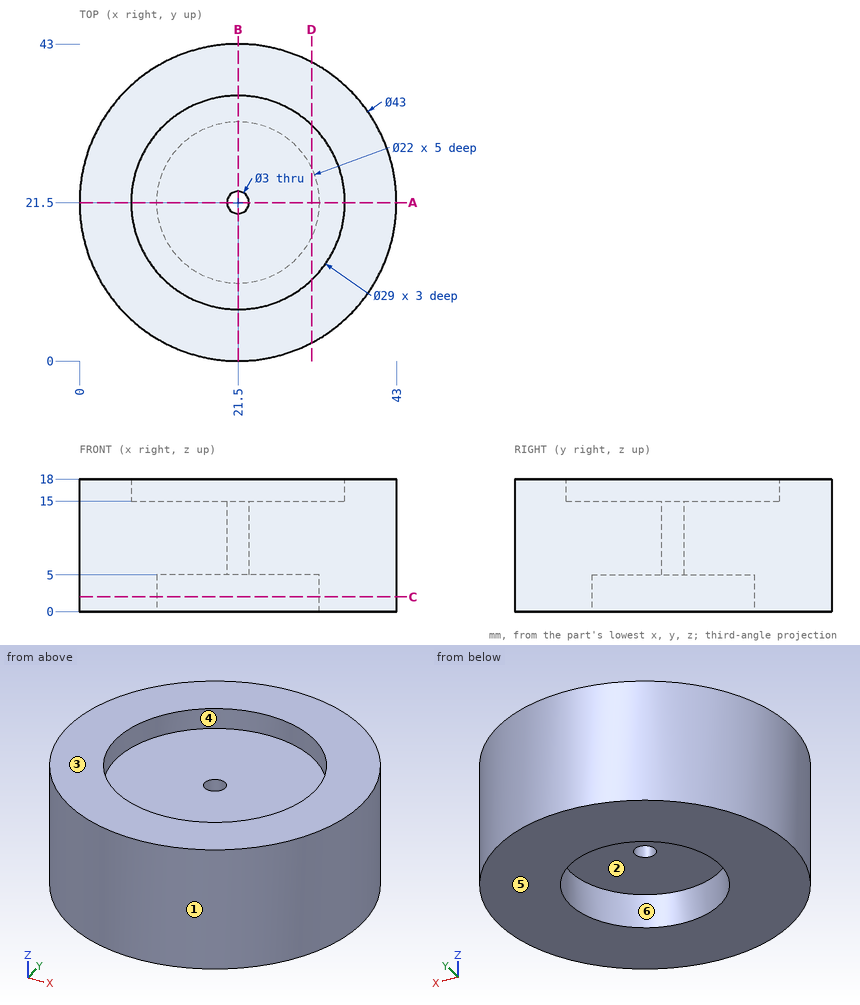
Here's the drawing with two shaded views (mm, measured from the low corner). I have some questions. A direction names the side the tool comes from. Coordinates: 2 decimals unless noted, no trailing zeros. Order: outer loops, then holes, each group sorted by start corner. A loop starts at its lowest first (then second) coordinate and runs counter-clockwise, first axis right, second up. Notation, with made-up numbers: (17, -39) - (50, -39) arc R17 ccw to (50, -15) - close; hole circle Ø1 at (44, 89). An arc over 180 degrees is marked (long way). Answer in a Markdown table with one row per item.
1. Suppose I cut it at D-D (x = 31.5). Please give me the cut outline in (y, z), and give its area (3 significant figures).
Reply:
| item | result |
|---|---|
| outline | (2.47, 0) - (16.92, 0) - (16.92, 5) - (26.08, 5) - (26.08, 0) - (40.53, 0) - (40.53, 18) - (32, 18) - (32, 15) - (11, 15) - (11, 18) - (2.47, 18) - close |
| area | 576 mm^2 |
2. Suppose I cut it at C-C (z = 2). Please give me the cut outline in (x, y).
Reply:
| item | result |
|---|---|
| outline | circle Ø43 at (21.5, 21.5); hole circle Ø22 at (21.5, 21.5) |
3. For the marked faces 4, 5 and 6, which set-ups out of +Z, -Z, +X, -X, +Y, -Y let a thin tool reach every point of the face, with its end or its side?
Reply:
| item | result |
|---|---|
| face 4 | +Z |
| face 5 | -Z, +X, -X, +Y, -Y |
| face 6 | -Z |
4. If we mould it in two halves opening along Y, with no side actions, what happens to the marked faces 1, 2 and 3? For each: pulls with the +Y half, pulls with the -Y half, needs draft (parallel to the pull), parting line crosses it, or undercut.
Reply:
| item | result |
|---|---|
| face 1 | parting line crosses it |
| face 2 | undercut |
| face 3 | needs draft |
5. If I drill on line 1 along Y through (x, z) = (21.5, 16.7); line 2 along Z through (x, y) = (16.5, 16); line 3 along X through (y, z) = (14, 1), over which ranges is the centre line in solid material (lowest first)?
Reply:
| item | result |
|---|---|
| line 1 | y = 0 to 7, 36 to 43 |
| line 2 | z = 5 to 15 |
| line 3 | x = 1.35 to 13.45, 29.55 to 41.65 |
6. For pin 1 (4 mm diameter, centred on x = 21.5, y = 21.5, fed in from -Z); pin 2 (5 mm diameter, centred on y = 35, z = 7.5, fed in from +X); pin 3 (5 mm diameter, centred on y = 13.5, z = 13, fed in from -X), each with a flat end and sliding along its axis, tell me the tip position at first contact or that it passes through.
Reply:
| item | result |
|---|---|
| pin 1 | stops at z = 5 |
| pin 2 | stops at x = 39.97 |
| pin 3 | stops at x = 0.72 |
7. Suppose I cut it at A-A (y = 21.5). Please give me the cut outline in (x, z), and give its area (3 significant figures).
Reply:
| item | result |
|---|---|
| outline | (0, 0) - (10.5, 0) - (10.5, 5) - (20, 5) - (20, 15) - (7, 15) - (7, 18) - (0, 18) - close; (23, 5) - (32.5, 5) - (32.5, 0) - (43, 0) - (43, 18) - (36, 18) - (36, 15) - (23, 15) - close |
| area | 547 mm^2 |
